Here's how the part is built. I have some questions about the finished solid (model axes, mm). Round coordinates to 2 decimals unless told otherwise and drop trailing zeros. Loops run counter-clockwise (first coordinate to the right, second up) from the corner with the lowest first, then second, coordinate; pieces in that order, holes last. Notation, with made-up numbers: M 57.5,79.5 L 89.5,79.5 A28 ccw 89.5,104.5 Z; hole C 28,32 d10. An arc over 180 degrees is marked long. Write each question's results on one line, items separated by ' | '. Start each with the question number.
```python
from build123d import *

# Parameters (mm, degrees)
SKETCH1_W           = 20
SKETCH1_H           = 20
SKETCH1_R           = 1.75
BOSS_EXTRUDE1_DEPTH = 2
CHAMFER1_SIZE       = 3


with BuildPart() as part:
    # Sketch1 → Boss-Extrude1 (new body)
    with BuildSketch(Plane(origin=(0, 0, 0), x_dir=(1, 0, 0), z_dir=(0, 1, 0))):
        Rectangle(SKETCH1_W, SKETCH1_H)
        with Locations(Location((0, 0, 0), (0, 0, 270))):
            Circle(SKETCH1_R, mode=Mode.SUBTRACT)
    extrude(amount=BOSS_EXTRUDE1_DEPTH)

    # Chamfer1
    chamfer1_edges = [part.edges().sort_by_distance(p)[0] for p in [
        (-10, 1, -10),
        (10, 1, -10),
        (10, 1, 10),
        (-10, 1, 10),
    ]]
    chamfer(chamfer1_edges, length=CHAMFER1_SIZE)


solid = part.part
```
1. If we mould it in two halves opening along Z, with no side actions, what happens to faces 1 (the face through (9, 1, 8)), 2 (the face through (-10, 1, 0)), 3 (the face through (-1.71, 0.99, -0.38))? For each: released by +Z, released by -Z, zero draft, split by the parting line, or undercut.
2. I want a section at A-A on x = 0. List the corners of the cut face in (y, z) for me.
3. I need wall thicknesses on line 1 along X through (y, z) = (0.75, 0); line 2 along Z through (x, y) = (1.25, 0.75); line 3 along Z through (x, y) = (0.75, 0.4). Which ranges of each line are inside material? Lowest first, please.
4. I want a section at D-D on z = -8. List the corners of the cut face in (x, y) for me, plus the area to 3 significant figures.
5. For pin 1 (1 mm diameter, centred on x = 8, y = 0.5, fed in from -Z), with a flat end and sliding along its axis, tell me the tip position at first contact or that it passes through.
6. I want a section at B-B on z = 0. List the corners of the cut face in (x, y) for me.
7. I want a section at C-C on y = 0.85. List the corners of the cut face in (x, z) for me, plus the area to 3 significant figures.
Outcome:
1) face 1: released by +Z | face 2: zero draft | face 3: undercut
2) outline: M 0,-10 L 2,-10 L 2,-1.75 L 0,-1.75 Z; M 0,1.75 L 2,1.75 L 2,10 L 0,10 Z
3) line 1: -10 to -1.75, 1.75 to 10 | line 2: -10 to -1.22, 1.22 to 10 | line 3: -10 to -1.58, 1.58 to 10
4) outline: M -9,0 L 9,0 L 9,2 L -9,2 Z | area: 36.0 mm2
5) pin 1: z = -9.5
6) outline: M -10,0 L -1.75,0 L -1.75,2 L -10,2 Z; M 1.75,0 L 10,0 L 10,2 L 1.75,2 Z
7) outline: M -10,-7 L -7,-10 L 7,-10 L 10,-7 L 10,7 L 7,10 L -7,10 L -10,7 Z; hole C 0,0 d3.5 | area: 372 mm2
